Here's how the part is built. I have some questions about the finished solid (model axes, mm). Face numbers are marked on the shaded views. A direction names the side the tool comes from. Round coordinates to 2 decimals unless told otherwise and drop trailing zeros. Loops run counter-clockwise (first coordinate to the right, second up) from the corner with the lowest first, then second, coordinate; pieces in that order, holes last. Notation, with made-up numbers: (23.5, 75) -> (30.5, 75) arc R18 ccw to (30.5, 85) -> close; hole circle Ø3 at (11.25, 56.25). An arc over 180 degrees is marked (long way). Use one line per item in the form item = value. Start each with the question number.
Item 1: For the marked faces 1 and 2, which set-ups out of +Z, -Z, +X, -X, +Y, -Y let a thin tool reach every point of the face, with its end or its side?
Item 2: If I drill on L1, parallel to Y at x = 0, z = 25.05; L2, parallel to Y at x = -0.5, z = 24.5; L3, parallel to Y at x = 5.5, z = 21, over which ranges is the centre line in solid material (lowest first)? Write a range as [from, to].
Item 3: If we section it at A-A (y = 6): Write out the boundary of the cut face in (x, z), then the cut area to 3 significant figures.
Item 4: I'm going to push flat-ended pins straight in: pin 1 Ø2 at (x, z) = (0, 0.55) entering from -Y; pin 2 Ø8.5 at (x, y) = (0, 14.5) entering from -Z; pin 3 Ø0.5 at (x, y) = (-11, 1) entering from +Z; pin 4 Ø4 at (x, z) = (0, -12.15) entering from +Y. Where does each tip first touch, or does it pass through?
Item 5: If we section it at C-C (y = 13.5): Write out the boundary of the cut face in (x, z).
Item 6: If we section it at D-D (x = 0): State how many separate pieces and enclosed holes the cut face has, then the cut area to 3 significant figures.
Item 7: If we section it at B-B (x = 7.5): Write out the boundary of the cut face in (y, z), then the cut area to 3 significant figures.
Autodesk Inventor part; units mm, degrees
ref_plane "YZ Plane" through (0, 0, 0) normal (1, 0, 0) x (0, 1, 0)
ref_plane "XZ Plane" through (0, 0, 0) normal (0, 1, 0) x (-1, 0, 0)
ref_plane "XY Plane" through (0, 0, 0) normal (0, 0, 1) x (1, 0, 0)
sketch "Sketch1" plane through (0, 0, 0) normal (0, 1, 0) x (-1, 0, 0)
  line L0 (-12.5, 26) -> (12.5, 26)
  line L1 (12.5, 26) -> (12.5, 19.2)
  line L2 (8.5, -26) -> (-8.5, -26)
  circle A0 centre (0, 19.6) radius 1.65
  line L3 (0, 26) -> (10.85, 26)
  arc A1 (10.85, 18.2) -> (10.85, 14.8) centre (10.85, 16.5) ccw
  line L4 (10.85, 18.2) -> (11.5, 18.2)
  line L5 (10.85, 14.8) -> (11.5, 14.8)
  arc A2 (11.5, 18.2) -> (12.5, 19.2) centre (11.5, 19.2) ccw
  arc A3 (12.5, 13.8) -> (11.5, 14.8) centre (11.5, 13.8) ccw
  arc A4 (10.85, 11.85) -> (10.85, 8.45) centre (10.85, 10.15) ccw
  line L6 (10.85, 11.85) -> (11.5, 11.85)
  line L7 (10.85, 8.45) -> (11.5, 8.45)
  arc A5 (11.5, 11.85) -> (12.5, 12.85) centre (11.5, 12.85) ccw
  arc A6 (12.5, 7.45) -> (11.5, 8.45) centre (11.5, 7.45) ccw
  arc A7 (10.85, 5.5) -> (10.85, 2.1) centre (10.85, 3.8) ccw
  line L8 (10.85, 5.5) -> (11.5, 5.5)
  line L9 (10.85, 2.1) -> (11.5, 2.1)
  arc A8 (11.5, 5.5) -> (12.5, 6.5) centre (11.5, 6.5) ccw
  arc A9 (12.5, 1.1) -> (11.5, 2.1) centre (11.5, 1.1) ccw
  arc A10 (10.85, -0.85) -> (10.85, -4.25) centre (10.85, -2.55) ccw
  line L10 (10.85, -0.85) -> (11.5, -0.85)
  line L11 (10.85, -4.25) -> (11.5, -4.25)
  arc A11 (11.5, -0.85) -> (12.5, 0.15) centre (11.5, 0.15) ccw
  arc A12 (12.5, -5.25) -> (11.5, -4.25) centre (11.5, -5.25) ccw
  arc A13 (10.85, -7.2) -> (10.85, -10.6) centre (10.85, -8.9) ccw
  line L12 (10.85, -7.2) -> (11.5, -7.2)
  line L13 (10.85, -10.6) -> (11.5, -10.6)
  arc A14 (11.5, -7.2) -> (12.5, -6.2) centre (11.5, -6.2) ccw
  arc A15 (12.5, -11.6) -> (11.5, -10.6) centre (11.5, -11.6) ccw
  arc A16 (10.85, -13.55) -> (10.85, -16.95) centre (10.85, -15.25) ccw
  line L14 (10.85, -13.55) -> (11.5, -13.55)
  line L15 (10.85, -16.95) -> (11.5, -16.95)
  arc A17 (11.5, -13.55) -> (12.5, -12.55) centre (11.5, -12.55) ccw
  arc A18 (12.5, -17.95) -> (11.5, -16.95) centre (11.5, -17.95) ccw
  line L16 (12.5, 13.8) -> (12.5, 12.85)
  line L17 (12.5, 7.45) -> (12.5, 6.5)
  line L18 (12.5, 1.1) -> (12.5, 0.15)
  line L19 (12.5, -5.25) -> (12.5, -6.2)
  line L20 (12.5, -11.6) -> (12.5, -12.55)
  line L21 (12.5, -17.95) -> (12.5, -22)
  line L22 (-12.5, 26) -> (-12.5, 19.2)
  arc A19 (-10.85, 14.8) -> (-10.85, 18.2) centre (-10.85, 16.5) ccw
  line L23 (-10.85, 18.2) -> (-11.5, 18.2)
  line L24 (-10.85, 14.8) -> (-11.5, 14.8)
  arc A20 (-12.5, 19.2) -> (-11.5, 18.2) centre (-11.5, 19.2) ccw
  arc A21 (-11.5, 14.8) -> (-12.5, 13.8) centre (-11.5, 13.8) ccw
  arc A22 (-11.5, 8.45) -> (-12.5, 7.45) centre (-11.5, 7.45) ccw
  line L25 (-10.85, 8.45) -> (-11.5, 8.45)
  line L26 (-10.85, 11.85) -> (-11.5, 11.85)
  arc A23 (-12.5, 12.85) -> (-11.5, 11.85) centre (-11.5, 12.85) ccw
  arc A24 (-10.85, 8.45) -> (-10.85, 11.85) centre (-10.85, 10.15) ccw
  arc A25 (-11.5, 2.1) -> (-12.5, 1.1) centre (-11.5, 1.1) ccw
  line L27 (-10.85, 2.1) -> (-11.5, 2.1)
  line L28 (-10.85, 5.5) -> (-11.5, 5.5)
  arc A26 (-12.5, 6.5) -> (-11.5, 5.5) centre (-11.5, 6.5) ccw
  arc A27 (-10.85, 2.1) -> (-10.85, 5.5) centre (-10.85, 3.8) ccw
  arc A28 (-11.5, -4.25) -> (-12.5, -5.25) centre (-11.5, -5.25) ccw
  line L29 (-10.85, -4.25) -> (-11.5, -4.25)
  line L30 (-10.85, -0.85) -> (-11.5, -0.85)
  arc A29 (-12.5, 0.15) -> (-11.5, -0.85) centre (-11.5, 0.15) ccw
  arc A30 (-10.85, -4.25) -> (-10.85, -0.85) centre (-10.85, -2.55) ccw
  arc A31 (-11.5, -10.6) -> (-12.5, -11.6) centre (-11.5, -11.6) ccw
  line L31 (-10.85, -10.6) -> (-11.5, -10.6)
  line L32 (-10.85, -7.2) -> (-11.5, -7.2)
  arc A32 (-12.5, -6.2) -> (-11.5, -7.2) centre (-11.5, -6.2) ccw
  arc A33 (-10.85, -10.6) -> (-10.85, -7.2) centre (-10.85, -8.9) ccw
  arc A34 (-11.5, -16.95) -> (-12.5, -17.95) centre (-11.5, -17.95) ccw
  line L33 (-10.85, -16.95) -> (-11.5, -16.95)
  line L34 (-10.85, -13.55) -> (-11.5, -13.55)
  arc A35 (-12.5, -12.55) -> (-11.5, -13.55) centre (-11.5, -12.55) ccw
  arc A36 (-10.85, -16.95) -> (-10.85, -13.55) centre (-10.85, -15.25) ccw
  line L35 (-12.5, 13.8) -> (-12.5, 12.85)
  line L36 (-12.5, 7.45) -> (-12.5, 6.5)
  line L37 (-12.5, 1.1) -> (-12.5, 0.15)
  line L38 (-12.5, -5.25) -> (-12.5, -6.2)
  line L39 (-12.5, -11.6) -> (-12.5, -12.55)
  line L40 (-12.5, -17.95) -> (-12.5, -22)
  arc A37 (8.5, -26) -> (12.5, -22) centre (8.5, -22) ccw
  arc A38 (-12.5, -22) -> (-8.5, -26) centre (-8.5, -22) ccw
  circle A39 centre (0, 13.25) radius 1.65
  circle A40 centre (0, 6.9) radius 1.65
  circle A41 centre (0, 0.55) radius 1.65
  circle A42 centre (0, -5.8) radius 1.65
  circle A43 centre (0, -12.15) radius 1.65
  circle A44 centre (0, -18.5) radius 1.65
  point P0 (-12.5, -26)
  point P1 (12.5, -26)
  point P2 (12.5, 14.8)
  point P3 (12.5, 8.45)
  point P4 (12.5, 2.1)
  point P5 (12.5, -4.25)
  point P6 (12.5, -10.6)
  point P7 (12.5, -16.95)
  point P8 (-12.5, 14.8)
  point P9 (-12.5, 8.45)
  point P10 (-12.5, 2.1)
  point P11 (-12.5, -4.25)
  point P12 (-12.5, -10.6)
  point P13 (-12.5, -16.95)
  dimension "d0" = 52
  dimension "d1" = 25
  dimension "d3" = 3.3
  dimension "d16" = 10.85
  dimension "d18" = 1.7
  dimension "d19" = 1
  dimension "d20" = 1
  dimension "d22" = 1.7
  dimension "d23" = 1
  dimension "d24" = 1
  dimension "d26" = 1.7
  dimension "d27" = 1
  dimension "d28" = 1
  dimension "d30" = 1.7
  dimension "d31" = 1
  dimension "d32" = 1
  dimension "d34" = 1.7
  dimension "d35" = 1
  dimension "d36" = 1
  dimension "d38" = 1.7
  dimension "d39" = 1
  dimension "d40" = 1
  dimension "d42" = 4
  dimension "d44" = 3.3
  dimension "d46" = 3.3
  dimension "d48" = 3.3
  dimension "d50" = 3.3
  dimension "d52" = 3.3
  dimension "d54" = 3.3
extrude "Extrusion1" add sketch "Sketch1" along normal blind 2
sketch "Sketch2" plane through (0, 2, 0) normal (0, 1, 0) x (1, 0, 0)
  line L0 (-12.5, -26) -> (12.5, -26)
  line L1 (12.5, -26) -> (12.5, -24)
  line L2 (12.5, -24) -> (-12.5, -24)
  line L3 (-12.5, -24) -> (-12.5, -26)
  point P0 (0, 0)
  dimension "d60" = 2
extrude "Extrusion2" add sketch "Sketch2" along normal blind 27
sketch "Sketch3" plane through (-12.5, 0, 26) normal (0, 0, 1) x (1, 0, 0)
  circle A0 centre (12.5, 14.5) radius 3.75
  circle A1 centre (12.5, 23) radius 1.65
  circle A2 centre (4, 14.5) radius 1.65
  circle A3 centre (12.5, 6) radius 1.65
  circle A4 centre (21, 14.5) radius 1.65
  line L0 (0, 0) -> (0, 29)
  arc A5 (25, 14.5) -> (0, 14.5) centre (12.5, 14.5) ccw
  line L1 (0, 14.5) -> (0, 29)
  line L2 (0, 29) -> (25, 29)
  line L3 (25, 29) -> (25, 14.5)
  point P0 (12.5, 0)
  dimension "d63" = 14.5
  dimension "d64" = 7.5
  dimension "d66" = 3.3
  dimension "d69" = 360
extrude "Extrusion3" cut sketch "Sketch3" against normal through all
fillet "Fillet1" radius 2 1 edges at (0, 0, 26)
properties part number "Motor Mount Bracket" material "Aluminum 6061-AHC"
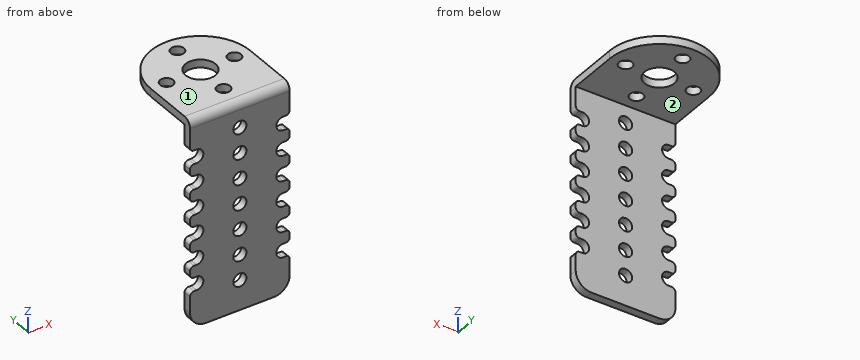
Values found:
q1.face_1 = +Z, +X, -X, +Y, -Y
q1.face_2 = -Z, +X, -X, +Y
q2.L1 = [0.3, 4.35], [7.65, 10.75], [18.25, 21.35], [24.65, 27]
q2.L2 = [0.06, 4.43], [7.57, 10.78], [18.22, 21.43], [24.57, 26.99]
q2.L3 = [0, 2]
q3.outline = (-12.5, 24) -> (-1.65, 24) -> (-1.65, 26) -> (-12.5, 26) -> close; (1.65, 24) -> (12.5, 24) -> (12.5, 26) -> (1.65, 26) -> close
q3.area = 43.4 mm2
q4.pin_1 = through
q4.pin_2 = 24
q4.pin_3 = 25.85
q4.pin_4 = 2
q5.outline = (-12.5, 24) -> (-9.81, 24) -> (-9.81, 26) -> (-12.5, 26) -> close; (-7.19, 24) -> (-3.61, 24) -> (-3.61, 26) -> (-7.19, 26) -> close; (3.61, 24) -> (7.19, 24) -> (7.19, 26) -> (3.61, 26) -> close; (9.81, 24) -> (12.5, 24) -> (12.5, 26) -> (9.81, 26) -> close
q6.separate_pieces = 11
q6.enclosed_holes = 0
q6.area = 78.7 mm2
q7.outline = (0, -26) -> (2, -26) -> (2, 24) -> (13.19, 24) -> (13.19, 26) -> (2, 26) arc R2 ccw to (0, 24) -> close; (15.81, 24) -> (24.5, 24) -> (24.5, 26) -> (15.81, 26) -> close
q7.area = 143 mm2
